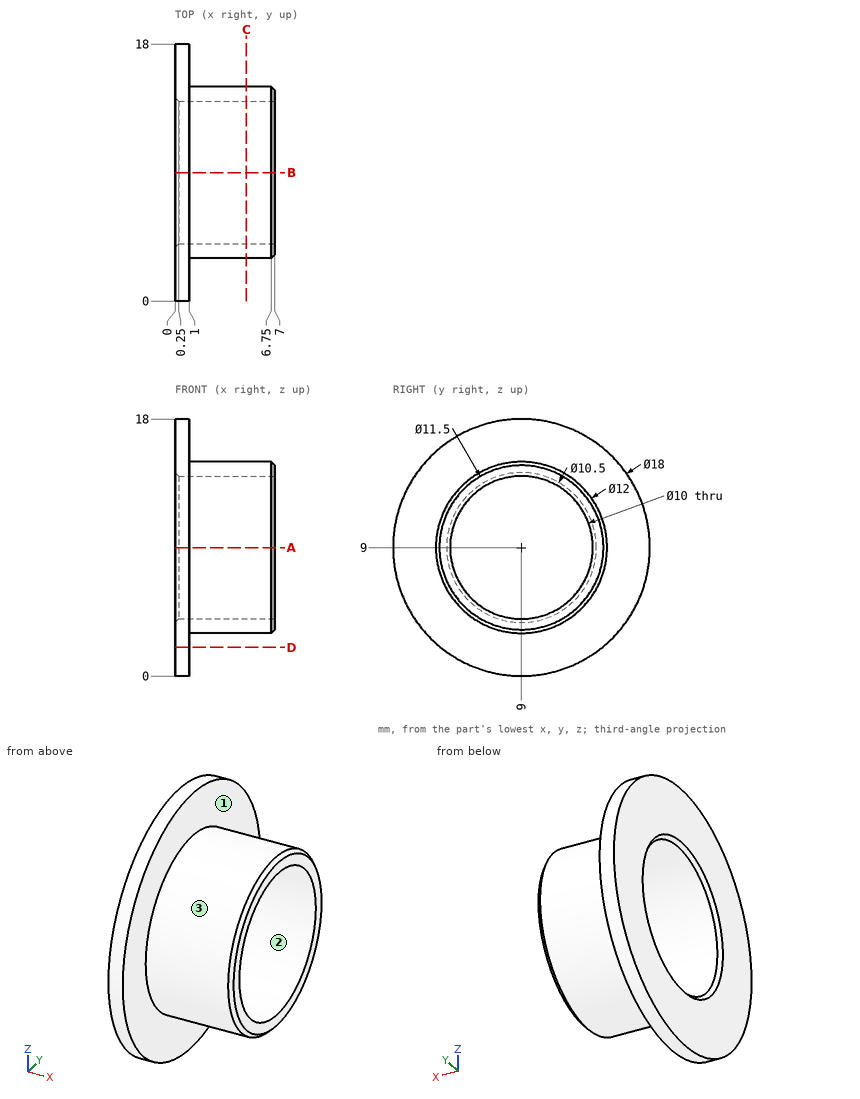
Geometry: see drawing. Coordinates: mm, zero at the bounding-box minimum. Give positions to 0.01 mm unless a question says otherwise; leave off trailing zeros. Write each loop counter-clockwise with the first axis right and the second up, starting at its lowest first coordinate (ties: lowest second). Pieces come first, ordered by that corner, then holes. Notation, with made-up numbers: M 86.5,37.25 L 117.5,37.25 A34 cw 117.5,72.25 Z; hole C 83,-8 d10. An arc over 180 degrees is marked long. Return JSON: item names as keys, results as strings. Group by question number.
1) Cut plane A-A, the plane z = 9. Output: boundary loops of the cut face in (x, y).
2) Cut plane D-D, the plane z = 2. Output: boundary loops of the cut face in (x, y).
3) Draft query along Y for the marked faces 1, 2 and 3. Return one class per face: released by +Y, released by -Y, zero draft, split by the parting line, or undercut.
4) Ray query, L1, parallel to Z at x = 5.25, y = 9; L2, parallel to X at y = 1.25, z = 8.75; L3, parallel to Y at x = 3.75, z = 9.5. Return the intervals inside material, ascending.
5) First-contact query: pin 1 Ø1 at (x, y) = (1, 15.5) entering from -Z; pin 2 Ø2 at (x, z) = (2.5, 15.5) entering from -Y; pin 3 Ø2 at (x, z) = (2.5, 15.5) entering from +Y. Flat tips, straight axial feed; report the tip coordinate or a pass-through.
6) Cut plane C-C, the plane x = 5. Output: boundary loops of the cut face in (y, z), then the cut area to 3 significant figures.
Data:
{
 "1": {"outline": "M 0,0 L 1,0 L 1,3 L 6.75,3 L 7,3.25 L 7,4 L 0.25,4 L 0,3.75 Z; M 0,14.25 L 0.25,14 L 7,14 L 7,14.75 L 6.75,15 L 1,15 L 1,18 L 0,18 Z"},
 "2": {"outline": "M 0,3.34 L 1,3.34 L 1,14.66 L 0,14.66 Z"},
 "3": {"face 1": "zero draft", "face 2": "undercut", "face 3": "split by the parting line"},
 "4": {"L1": "z = 3 to 4, 14 to 15", "L2": "x = 0 to 1", "L3": "y = 3.02 to 4.03, 13.97 to 14.98"},
 "5": {"pin 1": "stops at z = 2.29", "pin 2": "stops at y = 6.6", "pin 3": "stops at y = 11.4"},
 "6": {"outline": "C 9,9 d12; hole C 9,9 d10", "area": "34.6 mm²"}
}
